Input: dimensioned drawing with shaded views. Units: mm. Origin: part minimum x, y, z. Coordinates: 2 decimals unless noted, no trailing zeros. Loops run counter-clockwise (first coordinate to the right, second up) from the corner with the lowest first, then second, coordinate; pieces in that order, holes last.
(1) Line query: L1, parallel to Y at x = 5.5, z = 70; L2, parallel to Y at x = 6.75, z = 18.5 (1 decimal); L3, parallel to Z at x = 8, y = 103.5 (1 decimal). Output: solid intervals per line, ascending.
(2) Section A-A, the plane z = 70. Return loops of the section in (x, y), then the cut area to 3 significant figures.
(3) Section C-C, the plane z = 93. Return loops of the section in (x, y) (1 decimal).
(4) Mould query, pull axis Y, two halves, no side actions, for the marked faces 1, 2 and 3. Classes: released by +Y, released by -Y, zero draft, split by the parting line, or undercut.
(5) Section B-B, the plane y = 70. Return loops of the section in (x, z), then the cut area to 3 significant figures.
(6) Contact query for flat-ended pins moving along their axis: P1, Ø6, axis at x = 8, y = 112, coming from the -Z side; P2, Ø11, axis at y = 39.16, z = 17.55, coming from the -X side; P3, Ø21.5, axis at y = 130, z = 70, coming from the -X side; P4, Ø1.5, axis at x = 4.5, y = 59, coming from the -Z side (1 decimal). Output: stop coordinate, or through.
(7) Section D-D, the plane x = 5.25. Give the number of separate pieces and of enclosed holes in the cut face, then the cut area to 3 significant figures.
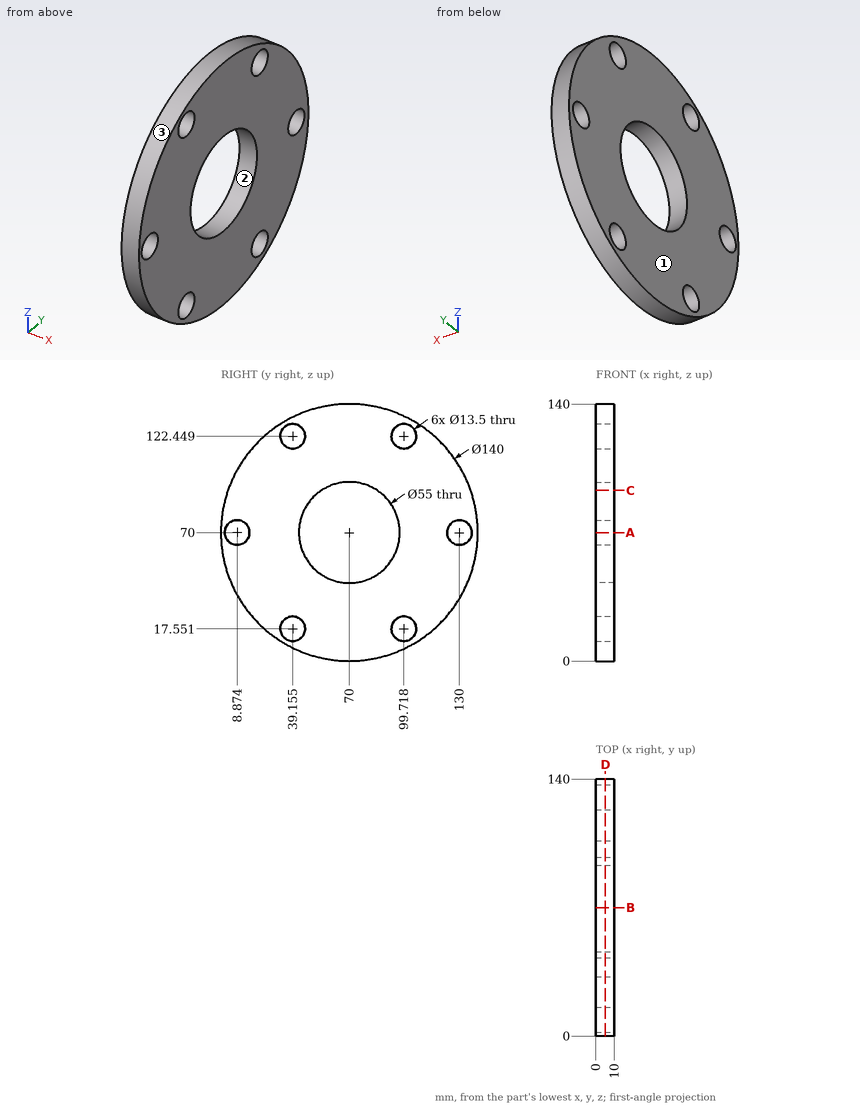
Report:
1. L1: y = 0 to 2.12, 15.62 to 42.5, 97.5 to 123.25, 136.75 to 140
1. L2: y = 22.6 to 32.5, 45.8 to 93, 106.4 to 117.4
1. L3: z = 8.5 to 12, 23.1 to 116.9, 128 to 131.5
2. outline: (0, 0) - (10, 0) - (10, 2.12) - (0, 2.12) - close; (0, 15.62) - (10, 15.62) - (10, 42.5) - (0, 42.5) - close; (0, 97.5) - (10, 97.5) - (10, 123.25) - (0, 123.25) - close; (0, 136.75) - (10, 136.75) - (10, 140) - (0, 140) - close
2. area: 580 mm2
3. outline: (0, 3.9) - (10, 3.9) - (10, 54.9) - (0, 54.9) - close; (0, 85.1) - (10, 85.1) - (10, 136.1) - (0, 136.1) - close
4. face 1: zero draft
4. face 2: undercut
4. face 3: split by the parting line
5. outline: (0, 0) - (10, 0) - (10, 42.5) - (0, 42.5) - close; (0, 97.5) - (10, 97.5) - (10, 140) - (0, 140) - close
5. area: 850 mm2
6. P1: stops at z = 11.87
6. P2: passes through
6. P3: stops at x = 0
6. P4: stops at z = 0.8
7. separate pieces: 1
7. enclosed holes: 7
7. area: 12,200 mm2
